from build123d import *

# Parameters (mm, degrees)
SKETCH1_W           = 108
SKETCH1_H           = 84
SKETCH1_R           = 2.25
SKETCH1_W_2         = 72
SKETCH1_H_2         = 72
BOSS_EXTRUDE1_DEPTH = 6.35
FILLET1_R           = 5


with BuildPart() as part:
    # Sketch1 → Boss-Extrude1 (new body)
    with BuildSketch(Plane.XY):
        with Locations((0.107594743, 0)):
            Rectangle(SKETCH1_W, SKETCH1_H)
        with Locations((-44.892405257, 30)):
            Circle(SKETCH1_R, mode=Mode.SUBTRACT)
        with Locations((45.107594743, 30)):
            Circle(SKETCH1_R, mode=Mode.SUBTRACT)
        with Locations((45.107594743, -30)):
            Circle(SKETCH1_R, mode=Mode.SUBTRACT)
        with Locations((-44.892405257, -30)):
            Circle(SKETCH1_R, mode=Mode.SUBTRACT)
        with Locations((0.107594743, 0)):
            Rectangle(SKETCH1_W_2, SKETCH1_H_2, mode=Mode.SUBTRACT)
    extrude(amount=BOSS_EXTRUDE1_DEPTH)

    # Fillet1
    fillet1_edges = [part.edges().sort_by_distance(p)[0] for p in [
        (-35.892405257, 36, 3.175),
        (-35.892405257, -36, 3.175),
        (36.107594743, -36, 3.175),
        (36.107594743, 36, 3.175),
        (-53.892405257, 42, 3.175),
        (54.107594743, 42, 3.175),
        (54.107594743, -42, 3.175),
        (-53.892405257, -42, 3.175),
    ]]
    fillet(fillet1_edges, radius=FILLET1_R)


solid = part.part
Read the model definition and answer for the solid it produces. Units are mm, in the model's axes. A direction names the side the tool comes from. Round coordinates to 2 decimals unless told otherwise and drop trailing zeros. Write each loop counter-clockwise with the first axis right and the second up, starting at its lowest first coordinate (ties: lowest second). Pieces come first, ordered by that corner, then holes. Notation, with made-up numbers: (33.5, 24.25) - (48.5, 24.25) arc R6 cw to (48.5, 29.25) - close; hole circle Ø4 at (-9, -17.75). An arc over 180 degrees is marked (long way). Use a Markdown table: item, result.
(1) The mould has two halves that part along Y. Classify faces 1 (the cylindrical face through (47.254, 30.676, 3.131)), 2 (the flat face through (-53.892, -1, 3)), 3 (the flat face through (-1, -42, 3)): released by +Y, released by -Y, zero draft, split by the parting line, or undercut.
Reported:
| item | result |
|---|---|
| face 1 | undercut |
| face 2 | zero draft |
| face 3 | released by -Y |
(2) The part is cut by section A-A (x = -23.5). Write down the section's boundary in (y, z), then the cut area to 3 significant figures.
Reported:
| item | result |
|---|---|
| outline | (-42, 0) - (-36, 0) - (-36, 6.35) - (-42, 6.35) - close; (36, 0) - (42, 0) - (42, 6.35) - (36, 6.35) - close |
| area | 76.2 mm2 |
(3) Which of the six approach directions +Z, -Z, +X, -X, +Y, -Y give full straight-line access (tool end or side, diameter ignored) to faces 4 (the cylindrical face through (-34.389, -34.574, 3.219)), 5 (the flat face through (-1, 42, 3))?
Reported:
| item | result |
|---|---|
| face 4 | +Z, -Z |
| face 5 | +Z, -Z, +X, -X, +Y |
(4) The part is cut by section B-B (y = -21). Write down the section's boundary in (x, z), then the cut area to 3 significant figures.
Reported:
| item | result |
|---|---|
| outline | (-53.89, 0) - (-35.89, 0) - (-35.89, 6.35) - (-53.89, 6.35) - close; (36.11, 0) - (54.11, 0) - (54.11, 6.35) - (36.11, 6.35) - close |
| area | 229 mm2 |
(5) This flat-tipped pin is pushed along its axis until it touches: pin 1 Ø4 at (x, y) = (-44.89, 30) entering from -Z. Where does it stop, or does it pass through?
Reported:
| item | result |
|---|---|
| pin 1 | through |
(6) The part is cut by section C-C (z = 3.5). Write down the section's boundary in (x, y), then the cut area to 3 significant figures.
Reported:
| item | result |
|---|---|
| outline | (-53.89, -37) arc R5 ccw to (-48.89, -42) - (49.11, -42) arc R5 ccw to (54.11, -37) - (54.11, 37) arc R5 ccw to (49.11, 42) - (-48.89, 42) arc R5 ccw to (-53.89, 37) - close; hole circle Ø4.5 at (-44.89, -30); hole circle Ø4.5 at (-44.89, 30); hole (-35.89, -31) arc R5 ccw to (-30.89, -36) - (31.11, -36) arc R5 ccw to (36.11, -31) - (36.11, 31) arc R5 ccw to (31.11, 36) - (-30.89, 36) arc R5 ccw to (-35.89, 31) - close; hole circle Ø4.5 at (45.11, -30); hole circle Ø4.5 at (45.11, 30) |
| area | 3,820 mm2 |
(7) The part is cut by section D-D (x = -45). Write down the section's boundary in (y, z), then the cut area to 3 significant figures.
Reported:
| item | result |
|---|---|
| outline | (-42, 0) - (-32.25, 0) - (-32.25, 6.35) - (-42, 6.35) - close; (-27.75, 0) - (27.75, 0) - (27.75, 6.35) - (-27.75, 6.35) - close; (32.25, 0) - (42, 0) - (42, 6.35) - (32.25, 6.35) - close |
| area | 476 mm2 |
(8) Straight lines are drawn through the part: line 1 along Y through (x, z) = (9, 4.75); line 2 along X through (y, z) = (-9, 2.5); line 3 along Y through (x, z) = (-45, 5.25). For each, find the intervals that lie inside material, in ascending order. Write a range as [from, to].
Reported:
| item | result |
|---|---|
| line 1 | [-42, -36], [36, 42] |
| line 2 | [-53.89, -35.89], [36.11, 54.11] |
| line 3 | [-42, -32.25], [-27.75, 27.75], [32.25, 42] |
